Input: part model. Units: mm. Frame: model coordinates. A direction names the side the tool comes from. Coordinates: 2 decimals unless noted, no trailing zeros. Order: outer loops, then holes, each group sorted by start corner. A loop starts at its lowest first (then second) coordinate and runs counter-clockwise, first axis right, second up.
from build123d import *

# Parameters (mm, degrees)
SKETCH1_W          = 114.3
SKETCH1_H          = 50.8
BASE_FLANGE1_DEPTH = 0.7
EDGE_FLANGE1_DEPTH = 114.3
EDGE_FLANGE2_DEPTH = 114.3


# Sheet-metal steps are written as plain solids
with BuildPart() as part:
    # Sketch1 → Base-Flange1 (new body)
    with BuildSketch(Plane(origin=(0, 0, 0), x_dir=(1, 0, 0), z_dir=(0, 1, 0))):
        Rectangle(SKETCH1_W, SKETCH1_H)
    extrude(amount=-BASE_FLANGE1_DEPTH)

    # Edge-Flange1 section (across the edge) → Edge-Flange1 (add)
    with BuildSketch(Plane(origin=(57.15, 0, -27.2), x_dir=(0, 0, 1), z_dir=(-1, 0, 0))):
        with BuildLine():
            Line((-0.7, 1), (-0.7, 152.4))
            Line((-0.7, 152.4), (0, 152.4))
            Line((0, 152.4), (0, 1))
            ThreePointArc((0, 1), (0.292893219, 0.292893219), (1, 0))
            Line((1, 0), (1.8, 0))
            Line((1.8, 0), (1.8, -0.7))
            Line((1.8, -0.7), (1, -0.7))
            ThreePointArc((1, -0.7), (-0.202081528, -0.202081528), (-0.7, 1))
        make_face()
    extrude(amount=EDGE_FLANGE1_DEPTH)

    # Edge-Flange2 section (across the edge) → Edge-Flange2 (add)
    with BuildSketch(Plane(origin=(57.15, 152.814213562, -27.2), x_dir=(0, -0.7071067811865414, 0.7071067811865537), z_dir=(-1, 0, 0))):
        with BuildLine():
            Line((-0.7, 0.414213562), (-0.7, 71.541250506))
            Line((-0.7, 71.541250506), (0, 71.541250506))
            Line((0, 71.541250506), (0, 0.414213562))
            ThreePointArc((0, 0.414213562), (0.076120467, 0.03153013), (0.292893219, -0.292893219))
            Line((0.292893219, -0.292893219), (-0.202081528, -0.787867966))
            ThreePointArc((-0.202081528, -0.787867966), (-0.570595205, -0.236348273), (-0.7, 0.414213562))
        make_face()
    extrude(amount=EDGE_FLANGE2_DEPTH)


solid = part.part
Item 1: Cut plane A-A on z = 11.5. Return loops of the section in (x, y), then the cut area to 3 significant figures.
Response values:
outline: (-57.15, -0.7) - (57.15, -0.7) - (57.15, 0) - (-57.15, 0) - close; (-57.15, 191.51) - (57.15, 191.51) - (57.15, 192.5) - (-57.15, 192.5) - close
area: 193 mm2
Item 2: Cut plane C-C on y = 14.5. Return loops of the section in (x, z).
Response values:
outline: (-57.15, -27.9) - (57.15, -27.9) - (57.15, -27.2) - (-57.15, -27.2) - close
Item 3: Cut plane B-B on x = -37.5. Return loops of the section in (y, z).
Response values:
outline: (-0.7, -26.2) arc R1.7 ccw to (1, -27.9) - (152.4, -27.9) arc R1.7 ccw to (153.6, -27.4) - (203.9, 22.89) - (203.4, 23.39) - (153.11, -26.91) arc R1 cw to (152.4, -27.2) - (1, -27.2) arc R1 cw to (0, -26.2) - (0, 25.4) - (-0.7, 25.4) - close
Item 4: Draft query along Y for faces 1 (the face through (1, 76, -27.9)), 2 (the face through (1, 78, -27.2)), 3 (the face through (0.8, 178.397, -2.607)), 4 (the face through (1, 0, -1)). Return one class per face: pulls with the +Y half, pulls with the -Y half, needs draft (parallel to the pull), parting line crosses it, or undercut.
Response values:
face 1: needs draft
face 2: undercut
face 3: pulls with the +Y half
face 4: undercut
Item 5: Pin query (flat end, axial travel): pin 1 Ø6 at (x, z) = (21.5, -7.5) entering from +Y; pin 2 Ø8 at (x, y) = (-39, 153.5) entering from -Z. Return the tip coordinate at first contact, or that it passes through.
Response values:
pin 1: stops at y = 176.5
pin 2: stops at z = -27.9
Item 6: Access query for faces 5 (the face through (1, -0.7, 0)), 6 (the face through (0.8, 178.606, -1.408)). Directions: +Z, -Z, +X, -X, +Y, -Y. A direction counts if a zero-diameter tool reaches every point of the face in a straight line with its end or side. Return the directions, or none.
Response values:
face 5: +Z, -Z, +X, -X, -Y
face 6: +Z, +X, -X
Item 7: Ray query, probe 1 along Y at (x, z) = (-31, -6.5); probe 2 along Y at (x, z) = (-0.5, -0.5); probe 3 along Y at (x, z) = (9.5, 23.5). Return the intervals inside material, ascending.
Response values:
probe 1: y = -0.7 to 0, 173.51 to 174.5
probe 2: y = -0.7 to 0, 179.51 to 180.5
probe 3: y = -0.7 to 0
